Work out the finished part from the listing and answer in its coordinate system (mm). Round coordinates to 2 decimals unless told otherwise and drop trailing zeros. Order: outer loops, then holes, each group sorted by start corner. A loop starts at its lowest first (then second) coordinate and runs counter-clockwise, first axis right, second up. Notation, with made-up numbers: (-5.5, 10.5) - (1.5, 10.5) arc R16 ccw to (1.5, 40.5) - close; hole circle Ø7 at (32, 3). An arc over 180 degrees is marked (long way). Put each result on its own line as item: value.
Autodesk Inventor part; units mm, degrees
ref_plane "YZ Plane" through (0, 0, 0) normal (1, 0, 0) x (0, 1, 0)
ref_plane "XZ Plane" through (0, 0, 0) normal (0, 1, 0) x (-1, 0, 0)
ref_plane "XY Plane" through (0, 0, 0) normal (0, 0, 1) x (1, 0, 0)
sketch "Sketch1" plane through (0, 0, 0) normal (0, 1, 0) x (-1, 0, 0)
  line L0 (49.034, 47.4336) -> (49.034, 46.8346)
  arc A0 (47.7204, 43.4566) -> (49.034, 46.8346) centre (44.034, 46.8346) ccw
  line L1 (47.7204, 43.4566) -> (36.3172, 31.0122)
  arc A1 (33.0666, 29.4092) -> (36.3172, 31.0122) centre (32.6308, 34.3902) ccw
  line L2 (33.0666, 29.4092) -> (-42.1497, 22.8286)
  arc A2 (-47.5855, 27.8096) -> (-42.1497, 22.8286) centre (-42.5855, 27.8096) ccw
  line L3 (-47.5855, 27.8096) -> (-47.5855, 34.3574)
  arc A3 (-37.5442, 45.3156) -> (-47.5855, 34.3574) centre (-36.5855, 34.3574) ccw
  line L4 (-37.5442, 45.3156) -> (43.5982, 52.4146)
  arc A4 (49.034, 47.4336) -> (43.5982, 52.4146) centre (44.034, 47.4336) ccw
  line L5 (35.9527, 27.654) -> (51.034, 44.1124)
  line L6 (51.034, 44.1124) -> (51.034, 55.0728)
  line L7 (51.034, 55.0728) -> (-37.7185, 47.308)
  arc A5 (-37.7185, 47.308) -> (-49.5855, 34.3574) centre (-36.5855, 34.3574) ccw
  line L8 (-49.5855, 34.3574) -> (-49.5855, 20.1704)
  line L9 (-49.5855, 20.1704) -> (35.9527, 27.654)
  line L10 (35.8578, 27.8465) -> (50.834, 44.1902)
  line L11 (50.834, 44.1902) -> (50.834, 54.8546)
  line L12 (50.834, 54.8546) -> (-37.7011, 47.1087)
  arc A6 (-37.7011, 47.1087) -> (-49.3855, 34.3574) centre (-36.5855, 34.3574) ccw
  line L13 (-49.3855, 34.3574) -> (-49.3855, 20.3887)
  line L14 (-49.3855, 20.3887) -> (35.8578, 27.8465)
  dimension "d0" = 0.2
extrude "Extrusion1" add sketch "Sketch1" along normal blind 0.4 contours L0 A0 L1 A1 L2 A2 L3 A3 L4 A4 | L9 L8 A5 L7 L6 L5 | L14 L13 A6 L12 L11 L10
properties part number "f"
1) A cutting plane is placed at B-B on z = 36.5. Write down the section's boundary in (x, y).
Findings below:
outline: (-44.06, 0) - (49.41, 0) - (49.41, 0.4) - (-44.06, 0.4) - close
2) A cutting plane is placed at A-A on y = 0.2. Write down the section's boundary in (x, z), then the cut area to 3 significant figures.
Findings below:
outline: (-51.03, 44.11) - (-35.95, 27.65) - (49.59, 20.17) - (49.59, 34.36) arc R13 ccw to (37.72, 47.31) - (-51.03, 55.07) - close
area: 2,480 mm2
3) Straight lines are drawn through the part: L1, parallel to X at y = 0.05, z = 32.5; L2, parallel to Z at x = -21, y = 0.3; L3, parallel to Z at x = -26.5, y = 0.3. For each, find the intervals that lie inside material, in ascending order. Write a range as from..to.
Findings below:
L1: x = -40.39..49.59
L2: z = 26.35..52.45
L3: z = 26.83..52.93
4) A cutting plane is placed at C-C on x = -15. Write down the section's boundary in (y, z).
Findings below:
outline: (0, 25.82) - (0.4, 25.82) - (0.4, 51.92) - (0, 51.92) - close
